```python
from build123d import *

# Parameters (mm, degrees)
F1_DEPTH  = 12.5
F3_DEPTH  = 25
F4_R      = 6.05
F5_DEPTH  = 55
F6_R      = 9.05
F7_DEPTH  = 52.5
F9_DEPTH  = 3
F11_DEPTH = 57.501
F13_DEPTH = 1


with BuildPart() as f1:
    # F0 (on Top) → F1 (new body, symmetric)
    with BuildSketch(Plane.XY):
        with BuildLine():
            ThreePointArc((50, 0), (0, -50), (-50, 0))
            Line((-50, 0), (-55, 0))
            ThreePointArc((-55, 0), (0, -55), (55, 0))
            Line((55, 0), (50, 0))
        make_face()
    extrude(amount=F1_DEPTH, both=True)

    # F2 (on face) → F3 (join)
    with BuildSketch(Plane.XY.offset(12.5)):
        with BuildLine():
            ThreePointArc((55, 0), (0, -55), (-55, 0))
            Line((-55, 0), (-55, -57.5))
            Line((-55, -57.5), (0, -57.5))
            Line((0, -57.5), (55, -57.5))
            Line((55, -57.5), (55, 0))
        make_face()
    extrude(amount=-F3_DEPTH)

    # F4 (on Front) → F5 (cut)
    with BuildSketch(Plane.XZ):
        Circle(F4_R)
    extrude(amount=F5_DEPTH, mode=Mode.SUBTRACT)

    # F6 (on Right) → F7 (cut, symmetric)
    with BuildSketch(Plane.YZ):
        with Locations((-11, 0)):
            Circle(F6_R)
    extrude(amount=F7_DEPTH, both=True, mode=Mode.SUBTRACT)

    # F8 (on face) → F9 (join)
    with BuildSketch(Plane.XZ.offset(57.5)):
        with BuildLine():
            Line((55, -1.825145), (56.187007, -1.825145))
            ThreePointArc((56.187007, -1.825145), (73.996764, 0.241309), (56.101841, 1.350101))
            Line((56.101841, 1.350101), (55, 1.350101))
            Line((55, 1.350101), (55, -1.825145))
        make_face()
        with BuildLine():
            Line((-55, 0.589209), (-56.019308, 0.589209))
            ThreePointArc((-56.019308, 0.589209), (-73.999691, -0.074534), (-56.010781, -0.440385))
            Line((-56.010781, -0.440385), (-55, -0.440385))
            Line((-55, -0.440385), (-55, 0.589209))
        make_face()
        with BuildLine():
            Line((26.665892, -12.5), (26.665892, -13.538735))
            ThreePointArc((26.665892, -13.538735), (27.491135, -31.499996), (28.35176, -13.540396))
            Line((28.35176, -13.540396), (28.35176, -12.5))
            Line((28.35176, -12.5), (26.665892, -12.5))
        make_face()
        with BuildLine():
            Line((-28.294771, -12.5), (-28.294771, -13.535161))
            ThreePointArc((-28.294771, -13.535161), (-27.521055, -31.499975), (-26.663293, -13.538978))
            Line((-26.663293, -13.538978), (-26.663293, -12.5))
            Line((-26.663293, -12.5), (-28.294771, -12.5))
        make_face()
        with BuildLine():
            Line((-26.327094, 12.5), (-26.327094, 13.576756))
            ThreePointArc((-26.327094, 13.576756), (-27.667739, 31.498437), (-28.339533, 13.539242))
            Line((-28.339533, 13.539242), (-28.339533, 12.5))
            Line((-28.339533, 12.5), (-26.327094, 12.5))
        make_face()
        with BuildLine():
            Line((28.639116, 12.5), (28.639116, 13.572379))
            ThreePointArc((28.639116, 13.572379), (27.368028, 31.499032), (26.623167, 13.542815))
            Line((26.623167, 13.542815), (26.623167, 12.5))
            Line((26.623167, 12.5), (28.639116, 12.5))
        make_face()
    extrude(amount=-F9_DEPTH)

    # F10 (on face) → F11 (cut, through all)
    with BuildSketch(Plane.XZ.offset(57.5)):
        Polygon((-15, 3), (-15, 12.5), (-15, 43.200534), (-80.149591, 43.200534), (-80.149591, -41.894257), (-15, -41.894257), (-15, -12.5), (-15, -3), (-21, -3), (-21, 0), (-21, 3), align=None)
        Polygon((15, 42.100117), (15, 12.5), (15, 3), (21, 3), (21, 0), (21, -3), (15, -3), (15, -12.5), (15, -47.119375), (79.776369, -47.119375), (79.776369, 42.100117), align=None)
    extrude(amount=-F11_DEPTH, mode=Mode.SUBTRACT)

    # F12 (on face) → F13 (join)
    with BuildSketch(Plane.XZ.offset(57.5)):
        with BuildLine():
            Line((-21, 0.785101), (-22.034309, 0.785101))
            ThreePointArc((-22.034309, 0.785101), (-39.999944, 0.031742), (-22.04007, -0.848323))
            Line((-22.04007, -0.848323), (-21, -0.848323))
            Line((-21, -0.848323), (-21, 0.785101))
        make_face()
        with BuildLine():
            Line((21, -0.86237), (22.041411, -0.86237))
            ThreePointArc((22.041411, -0.86237), (39.99991, 0.040222), (22.034061, 0.782262))
            Line((22.034061, 0.782262), (21, 0.782262))
            Line((21, 0.782262), (21, -0.86237))
        make_face()
    extrude(amount=-F13_DEPTH)


solid = f1.part
```
The model under review builds one solid part; all positions refer to its coordinate system, in mm. A direction names the side the tool comes from. Give positions to 0.01 mm unless a question says otherwise; leave off trailing zeros. Write each loop counter-clockwise with the first axis right and the second up, starting at its lowest first coordinate (ties: lowest second). Pieces come first, ordered by that corner, then holes. Notation, with made-up numbers: (86.25, 25.25) -> (91.25, 25.25) arc R13 cw to (91.25, 33.25) -> close; hole circle Ø11 at (38.5, 57). An arc over 180 degrees is marked (long way). Answer in a Markdown table with one row per item.
1) Add section B-B on x = 0. State the section outline as (y, z) points.
Worked answers:
| item | result |
|---|---|
| outline | (-57.5, -12.5) -> (-50, -12.5) -> (-50, -6.05) -> (-55, -6.05) -> (-55, 6.05) -> (-50, 6.05) -> (-50, 12.5) -> (-57.5, 12.5) -> close |
2) Add section C-C on z = 0. State the section outline as (x, y) points.
Worked answers:
| item | result |
|---|---|
| outline | (-40, -57.5) -> (40, -57.5) -> (40, -56.5) -> (21, -56.5) -> (21, -45.38) arc R50 cw to (6.05, -49.63) -> (6.05, -55) -> (-6.05, -55) -> (-6.05, -49.63) arc R50 cw to (-21, -45.38) -> (-21, -56.5) -> (-40, -56.5) -> close |
3) Add section D-D on z = -6.75. State the section outline as (x, y) points.
Worked answers:
| item | result |
|---|---|
| outline | (-36.95, -57.5) -> (-25.05, -57.5) -> (-25.05, -56.5) -> (-36.95, -56.5) -> close; (-15, -57.5) -> (15, -57.5) -> (15, -47.7) arc R50 cw to (-15, -47.7) -> close; (25.05, -57.5) -> (36.95, -57.5) -> (36.95, -56.5) -> (25.05, -56.5) -> close |
4) Add section A-A on y = -54.25. State the section outline as (x, z) points, plus the area to 3 significant figures.
Worked answers:
| item | result |
|---|---|
| outline | (-21, -3) -> (-15, -3) -> (-15, -12.5) -> (15, -12.5) -> (15, -3) -> (21, -3) -> (21, 3) -> (15, 3) -> (15, 12.5) -> (-15, 12.5) -> (-15, 3) -> (-21, 3) -> close; hole circle Ø12.1 at (0, 0) |
| area | 707 mm² |
5) For L1, parallel to Z at x = 0, y = -52.95; L2, parallel to Y at x = -0.5, z = -6.25; L3, parallel to X at y = -50.5, z = -6.5, list the stretches that pass through material, from the lowest coordinate up. Write a range as [from, to].
Worked answers:
| item | result |
|---|---|
| L1 | [-12.5, -6.05], [6.05, 12.5] |
| L2 | [-57.5, -50] |
| L3 | [-15, 15] |
6) Tool access review of faces 1 (the flat face through (18, -52, 3)), 2 (the flat face through (30, -56.5, 0)): name each direction out of +Z, -Z, +X, -X, +Y, -Y from which nothing blocks a thin tool from reaching the whole face with its end or side.
Worked answers:
| item | result |
|---|---|
| face 1 | +Z, +Y, -Y |
| face 2 | +Z, -Z, +X, +Y |
7) Clearance check with flat-ended pins moving along their axes: P1, Ø9, axis at x = 26, z = -4.5, coming from the +Y side; P2, Ø1.8, axis at x = 17.5, y = -49.5, coming from the +Z side; P3, Ø1, axis at y = -47.5, z = -7.5, coming from the +X side. State where each tip first meets the part, or that it passes through.
Worked answers:
| item | result |
|---|---|
| P1 | y = -56.5 |
| P2 | z = 3 |
| P3 | x = 15 |
8) Mouldability with a two-part tool opening along X and no side actions: class faces 3 (the flat face through (-31, -56.5, 0)), 4 (the cylindrical face through (-40, -57, 0)) as +X half, -X half, draft (parallel to the pull), parting line (faces both ways), or undercut.
Worked answers:
| item | result |
|---|---|
| face 3 | draft |
| face 4 | undercut |
